```python
from build123d import *

# Parameters (mm, degrees)
SKETCH1_W               = 24
SKETCH1_H               = 65
BOSS_EXTRUDE1_DEPTH     = 1.5
SKETCH2_W               = 12
SKETCH2_H               = 3
BOSS_EXTRUDE2_DEPTH     = 1.5
SKETCH4_W               = 3
SKETCH4_H               = 25
CUT_EXTRUDE1_DEPTH      = 2.5
CUT_EXTRUDE1_DEPTH_BACK = 2.5
FILLET1_R               = 3
SKETCH5_W               = 6
SKETCH5_H               = 3
CUT_EXTRUDE2_DEPTH      = 2.5
CUT_EXTRUDE2_DEPTH_BACK = 2.5


with BuildPart() as part:
    # Sketch1 → Boss-Extrude1 (new body, symmetric)
    with BuildSketch(Plane(origin=(0, 0, 0), x_dir=(1, 0, 0), z_dir=(0, 1, 0))):
        Rectangle(SKETCH1_W, SKETCH1_H)
    extrude(amount=BOSS_EXTRUDE1_DEPTH, both=True)

    # Sketch2 → Boss-Extrude2 (add, symmetric)
    with BuildSketch(Plane(origin=(0, 0, 0), x_dir=(1, 0, 0), z_dir=(0, 1, 0))):
        with Locations((0, -34)):
            Rectangle(SKETCH2_W, SKETCH2_H)
    extrude(amount=BOSS_EXTRUDE2_DEPTH, both=True)

    # Sketch4 → Cut-Extrude1 (cut, two sides)
    with BuildSketch(Plane(origin=(0, 0, 0), x_dir=(1, 0, 0), z_dir=(0, 1, 0))) as cut_extrude1_sk:
        with Locations((-7.5, 0)):
            Rectangle(SKETCH4_W, SKETCH4_H)
        with Locations((7.5, 0)):
            Rectangle(SKETCH4_W, SKETCH4_H)
    extrude(amount=CUT_EXTRUDE1_DEPTH, mode=Mode.SUBTRACT)
    extrude(cut_extrude1_sk.sketch, amount=-CUT_EXTRUDE1_DEPTH_BACK, mode=Mode.SUBTRACT)

    # Fillet1
    fillet1_edges = [part.edges().sort_by_distance(p)[0] for p in [
        (-12, 0, -32.5),
        (12, 0, -32.5),
    ]]
    fillet(fillet1_edges, radius=FILLET1_R)

    # Sketch5 → Cut-Extrude2 (cut, two sides)
    with BuildSketch(Plane(origin=(0, 0, 0), x_dir=(1, 0, 0), z_dir=(0, 1, 0))) as cut_extrude2_sk:
        with Locations((0, 31)):
            Rectangle(SKETCH5_W, SKETCH5_H)
    extrude(amount=CUT_EXTRUDE2_DEPTH, mode=Mode.SUBTRACT)
    extrude(cut_extrude2_sk.sketch, amount=-CUT_EXTRUDE2_DEPTH_BACK, mode=Mode.SUBTRACT)


solid = part.part
```
Read the model definition and answer for the solid it produces. Units are mm, in the model's axes. A direction names the side the tool comes from. Give positions to 0.01 mm unless a question says otherwise; leave off trailing zeros. Write each loop counter-clockwise with the first axis right and the second up, starting at its lowest first coordinate (ties: lowest second). Pieces come first, ordered by that corner, then holes. Notation, with made-up numbers: (52, 22.25) -> (89, 22.25) arc R19 cw to (89, 32.25) -> close; hole circle Ø3 at (-14, 1.25). An arc over 180 degrees is marked (long way). Answer as a JSON object with one key per item and string values.
1) Straight lines are drawn through the part: probe 1 along X at (y, z) = (0.9, 10); probe 2 along Z at (x, y) = (8, 0.95); probe 3 along Z at (x, y) = (-0.5, -1.1). For each, find the intervals that lie inside material, in ascending order. Write a range as from..to.
Findings below:
{"probe 1": "x = -12..-9, -6..6, 9..12", "probe 2": "z = -32.5..-12.5, 12.5..32.5", "probe 3": "z = -29.5..35.5"}
2) Section D-D on x = -1.5 is taken. Write down the section's boundary in (y, z).
Findings below:
{"outline": "(-1.5, -29.5) -> (1.5, -29.5) -> (1.5, 35.5) -> (-1.5, 35.5) -> close"}
3) Section B-B on x = -8.25 is taken. Write down the section's boundary in (y, z), then the cut area to 3 significant figures.
Findings below:
{"outline": "(-1.5, -32.5) -> (1.5, -32.5) -> (1.5, -12.5) -> (-1.5, -12.5) -> close; (-1.5, 12.5) -> (1.5, 12.5) -> (1.5, 32.5) -> (-1.5, 32.5) -> close", "area": "120 mm^2"}
4) Section A-A on z = 8 is taken. Write down the section's boundary in (x, y).
Findings below:
{"outline": "(-12, -1.5) -> (-9, -1.5) -> (-9, 1.5) -> (-12, 1.5) -> close; (-6, -1.5) -> (6, -1.5) -> (6, 1.5) -> (-6, 1.5) -> close; (9, -1.5) -> (12, -1.5) -> (12, 1.5) -> (9, 1.5) -> close"}
5) A tool of negligible diameter and unlimited length cuts with its end or side. For faces 5 (the flat face through (9, 0, 0)), 6 (the flat face through (0, 0, -29.5)), 7 (the flat face through (-6, 0, 34)), from which of +Z, -Z, +X, -X, +Y, -Y can it reach the whole face along a straight path? Write none if from no direction.
Findings below:
{"face 5": "+Y, -Y", "face 6": "-Z, +Y, -Y", "face 7": "+Z, -X, +Y, -Y"}
6) For a pull along X with two mould halves and no side action, classify faces 1 (the flat face through (6, 0, 0)), 2 (the flat face through (6, 0, 34)), 3 (the flat face through (9, 0, 32.5)), 4 (the flat face through (7, 0, 12.5)) as pulls with the +X half, pulls with the -X half, needs draft (parallel to the pull), parting line crosses it, or undercut.
Findings below:
{"face 1": "undercut", "face 2": "pulls with the +X half", "face 3": "needs draft", "face 4": "undercut"}
7) Section C-C on y = -0.8 is taken. Write down the section's boundary in (x, z), then the cut area to 3 significant figures.
Findings below:
{"outline": "(-12, -29.5) arc R3 ccw to (-9, -32.5) -> (-3, -32.5) -> (-3, -29.5) -> (3, -29.5) -> (3, -32.5) -> (9, -32.5) arc R3 ccw to (12, -29.5) -> (12, 32.5) -> (6, 32.5) -> (6, 35.5) -> (-6, 35.5) -> (-6, 32.5) -> (-12, 32.5) -> close; hole (-9, -12.5) -> (-6, -12.5) -> (-6, 12.5) -> (-9, 12.5) -> close; hole (6, -12.5) -> (9, -12.5) -> (9, 12.5) -> (6, 12.5) -> close", "area": "1,420 mm^2"}
